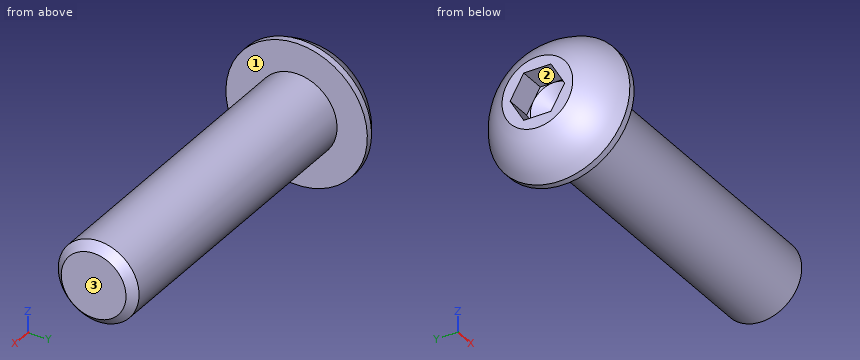
```python
from build123d import *

# Parameters (mm, degrees)
HEX_2_DEPTH = 3.0988


with BuildPart() as part:
    # BodySke → BaseBody (revolve)
    with BuildSketch(Plane.XY, mode=Mode.PRIVATE) as basebody_sk:
        with BuildLine():
            Line((42.9768, 0), (42.9768, 3.81635))
            Line((42.9768, 3.81635), (42.03065, 4.7625))
            Line((42.03065, 4.7625), (4.8768, 4.7625))
            Line((4.8768, 4.7625), (4.8768, 8.3312))
            Line((4.8768, 8.3312), (4.0894, 8.3312))
            ThreePointArc((4.0894, 8.3312), (1.712581673, 6.574442992), (0, 4.1656))
            Line((0, 4.1656), (0, 0))
            Line((0, 0), (42.9768, 0))
        make_face()
    revolve(basebody_sk.sketch.rotate(Axis((0, 0, 0), (1, 0, 0)), 90), axis=Axis((0, 0, 0), (1, 0, 0)))  # turned: the seam where the file's is

    # Sketch2 → PreBroach (revolve, cut)
    with BuildSketch(Plane.XY, mode=Mode.PRIVATE) as prebroach_sk:
        Polygon((0, 2.7813), (3.0988, 2.7813), (4.704584304, 0), (0, 0), align=None)
    revolve(prebroach_sk.sketch.rotate(Axis((0, 0, 0), (1, 0, 0)), 90), axis=Axis((0, 0, 0), (1, 0, 0)), mode=Mode.SUBTRACT)  # turned: the seam where the file's is

    # Sketch3 → Hex 2 (cut)
    with BuildSketch(Plane(origin=(0, 0, 0), x_dir=(0, 0, -1), z_dir=(1, 0, 0))):
        Polygon((-2.7813, -1.605784304), (-2.7813, 1.605784304), (0, 3.211568607), (2.7813, 1.605784304), (2.7813, -1.605784304), (0, -3.211568607), align=None)
    extrude(amount=HEX_2_DEPTH, mode=Mode.SUBTRACT)


solid = part.part
```
Geometry check sheet. Reference: the model listing, model coordinates, mm. Face numbers are marked on the shaded views. A direction names the side the tool comes from. Coordinates: 2 decimals unless noted, no trailing zeros. Write each loop counter-clockwise with the first axis right and the second up, starting at its lowest first coordinate (ties: lowest second). Pieces come first, ordered by that corner, then holes. Notation, with made-up numbers: M 25.25,9 L 58.25,9 A23 cw 58.25,25 Z; hole C 8.25,-36.5 d9. An arc over 180 degrees is marked long. Answer as a JSON object with one key per item and string values.
1. Scan lines: L1, parallel to Y at x = 35, z = -0.25; L2, parallel to X at y = -1.5, z = -0.25; L3, parallel to X at y = 1.75, z = 7.75. Record each from-to range of solid material in increasing order.
Answers below:
{"L1": "y = -4.76 to 4.76", "L2": "x = 3.83 to 42.98", "L3": "x = 3.41 to 4.88"}
2. Section check A-A, the plane x = 30. Enter the section's corners in (y, z) (1 decimal), plus the area to 3 significant figures.
Answers below:
{"outline": "C 0,0 d9.5", "area": "71.3 mm²"}
3. Tool access check on the marked faces 1, 2 and 3. Record the directions out of +Z, -Z, +X, -X, +Y, -Y that give a thin tool (end or side, any length) a straight path to the whole face; none if there is none.
Answers below:
{"face 1": "+X", "face 2": "-X", "face 3": "+Z, -Z, +X, +Y, -Y"}
4. Go/stop test with flat-tipped pins: pin 1 Ø1 at (x, z) = (34.5, 0) entering from +Y; pin 2 Ø2 at (y, z) = (-5.5, -6.5) entering from +X; pin 3 Ø1.5 at (y, z) = (-1, -2) entering from -X; pin 4 Ø5 at (y, z) = (-4, -0.5) entering from +X. Record where each tip stops, or that it passes through.
Answers below:
{"pin 1": "stops at y = 4.76", "pin 2": "stops at x = 4.88", "pin 3": "stops at x = 3.1", "pin 4": "stops at x = 42.98"}
